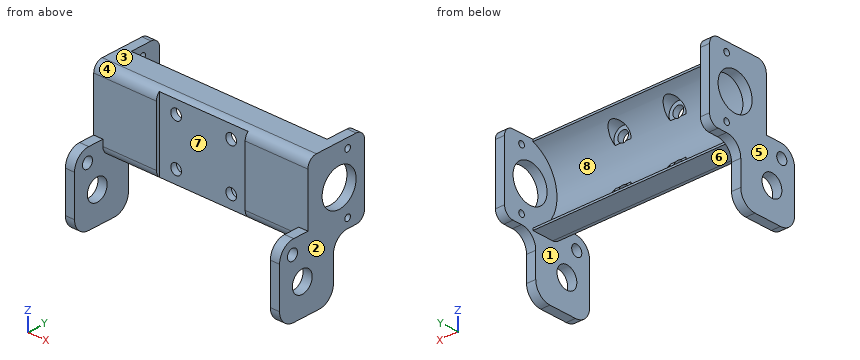
```python
from build123d import *

# Parameters (mm, degrees)
SKETCH1_W            = 70
SKETCH1_H            = 25
BOSS_EXTRUDE1_DEPTH  = 10
SKETCH2_W            = 3
SKETCH2_H            = 25
BOSS_EXTRUDE2_DEPTH  = 10
SKETCH3_R            = 12.5
CUT_EXTRUDE1_DEPTH   = 67
SKETCH4_R            = 3
CUT_EXTRUDE2_DEPTH   = 41.868692174
SKETCH5_R            = 1.75
CUT_EXTRUDE3_DEPTH   = 41.868692259
SKETCH6_W            = 29
SKETCH6_H            = 13
CUT_EXTRUDE4_DEPTH   = 1
SKETCH9_W            = 25
SKETCH9_H            = 20
BOSS_EXTRUDE3_DEPTH  = 3
SKETCH8_R            = 6
SKETCH8_R_2          = 1
CUT_EXTRUDE6_DEPTH   = 74.866433513
FILLET1_R            = 3
SKETCH10_W           = 23
SKETCH10_H           = 19
BOSS_EXTRUDE4_DEPTH  = 3
FILLET2_R            = 5
SKETCH11_R           = 3.5
CUT_EXTRUDE7_DEPTH   = 79.931932702
FILLET2_OF_MIRROR2_R = 5
FILLET3_R            = 5
FILLET4_R            = 3
SKETCH12_R           = 1.784400781
CUT_EXTRUDE8_DEPTH   = 79.931932702


# Some blends are built 0.0001 mm under size
with BuildPart() as part:
    # Sketch1 → Boss-Extrude1 (new body)
    with BuildSketch(Plane(origin=(0, 0, 0), x_dir=(1, 0, 0), z_dir=(0, 1, 0))):
        Rectangle(SKETCH1_W, SKETCH1_H)
    extrude(amount=BOSS_EXTRUDE1_DEPTH)

    # Sketch2 → Boss-Extrude2 (add)
    with BuildSketch(Plane(origin=(0, 10, 0), x_dir=(1, 0, 0), z_dir=(0, 1, 0))):
        with Locations((-33.5, 0)):
            Rectangle(SKETCH2_W, SKETCH2_H)
    extrude(amount=BOSS_EXTRUDE2_DEPTH)

    # Sketch3 → Cut-Extrude1 (cut)
    with BuildSketch(Plane(origin=(35, 0, 0), x_dir=(0, 0, -1), z_dir=(1, 0, 0))):
        with Locations((0, 14)):
            Circle(SKETCH3_R)
    extrude(amount=-CUT_EXTRUDE1_DEPTH, mode=Mode.SUBTRACT)

    # Sketch4 → Cut-Extrude2 (cut, through all)
    with BuildSketch(Plane(origin=(0, 3, 0), x_dir=(1, 0, 0), z_dir=(0, 1, 0))):
        with Locations((-9, 7.5)):
            Circle(SKETCH4_R)
        with Locations((9, 7.5)):
            Circle(SKETCH4_R)
    cut_extrude2 = extrude(amount=CUT_EXTRUDE2_DEPTH, mode=Mode.SUBTRACT)

    # Sketch5 → Cut-Extrude3 (cut, through all)
    with BuildSketch(Plane(origin=(0, 3, 0), x_dir=(1, 0, 0), z_dir=(0, 1, 0))):
        with Locations(Location((-9, 7.5, 0), (0, 0, 270))):
            Circle(SKETCH5_R)
        with Locations(Location((9, 7.5, 0), (0, 0, 270))):
            Circle(SKETCH5_R)
    cut_extrude3 = extrude(amount=-CUT_EXTRUDE3_DEPTH, mode=Mode.SUBTRACT)

    # Sketch6 → Cut-Extrude4 (cut)
    with BuildSketch(Plane.XZ):
        with Locations((0, -6)):
            Rectangle(SKETCH6_W, SKETCH6_H)
    cut_extrude4 = extrude(amount=-CUT_EXTRUDE4_DEPTH, mode=Mode.SUBTRACT)

    # Mirror1: Cut-Extrude2, Cut-Extrude3, Cut-Extrude4 across plane
    add(cut_extrude2.mirror(Plane.XY), mode=Mode.SUBTRACT)
    add(cut_extrude3.mirror(Plane.XY), mode=Mode.SUBTRACT)
    add(cut_extrude4.mirror(Plane.XY), mode=Mode.SUBTRACT)

    # Sketch9 → Boss-Extrude3 (add)
    with BuildSketch(Plane(origin=(35, 0, 0), x_dir=(0, 0, -1), z_dir=(1, 0, 0))):
        with Locations((0, 10)):
            Rectangle(SKETCH9_W, SKETCH9_H)
    extrude(amount=-BOSS_EXTRUDE3_DEPTH)

    # Sketch8 → Cut-Extrude6 (cut, through all)
    with BuildSketch(Plane.ZY.offset(35)):
        with Locations((0, 11)):
            Circle(SKETCH8_R)
        with Locations((-9.5, 14)):
            Circle(SKETCH8_R_2)
        with Locations((9.5, 14)):
            Circle(SKETCH8_R_2)
    extrude(amount=-CUT_EXTRUDE6_DEPTH, mode=Mode.SUBTRACT)

    # Fillet1
    fillet1_edges = [part.edges().sort_by_distance(p)[0] for p in [
        (33.5, 20, 12.5),
        (33.5, 20, -12.5),
        (-33.5, 20, 12.5),
        (-33.5, 20, -12.5),
    ]]
    fillet(fillet1_edges, radius=FILLET1_R)

    # Sketch10 → Boss-Extrude4 (add)
    with BuildSketch(Plane(origin=(35, 0, 0), x_dir=(0, 0, -1), z_dir=(1, 0, 0))):
        with Locations((19, -0.5)):
            Rectangle(SKETCH10_W, SKETCH10_H)
    boss_extrude4 = extrude(amount=-BOSS_EXTRUDE4_DEPTH)

    # Fillet2
    fillet2_edges = [part.edges().sort_by_distance(p)[0] for p in [
        (33.5, -10, -7.5),
        (33.5, 9, -30.5),
        (33.5, -10, -30.5),
    ]]
    fillet(fillet2_edges, radius=FILLET2_R)

    # Sketch11 → Cut-Extrude7 (cut, through all)
    with BuildSketch(Plane(origin=(35, 0, 0), x_dir=(0, 0, -1), z_dir=(1, 0, 0))):
        with Locations((20.5, -2)):
            Circle(SKETCH11_R)
    cut_extrude7 = extrude(amount=-CUT_EXTRUDE7_DEPTH, mode=Mode.SUBTRACT)

    # Mirror2: Boss-Extrude4, Cut-Extrude7 across plane
    add(boss_extrude4.mirror(Plane(origin=(0, 0, 0), x_dir=(0, 0, 1), z_dir=(1, 0, 0))))
    add(cut_extrude7.mirror(Plane(origin=(0, 0, 0), x_dir=(0, 0, 1), z_dir=(1, 0, 0))), mode=Mode.SUBTRACT)

    # Fillet2 of Mirror2
    fillet2_of_mirror2_edges = [part.edges().sort_by_distance(p)[0] for p in [
        (-33.5, -10, -7.5),
        (-33.5, 9, -30.5),
        (-33.5, -10, -30.5),
    ]]
    fillet(fillet2_of_mirror2_edges, radius=FILLET2_OF_MIRROR2_R)

    # Fillet3
    # the kernel refuses this fillet: 5 mm, written as the material it adds along each edge
    with BuildSketch(Plane(origin=(35, 9, -12.5), x_dir=(0, 1, 0), z_dir=(-1, 0, 0)), Plane(origin=(-35, 9, -12.5), x_dir=(0, 0, -1), z_dir=(1, 0, 0))) as fillet3_piece_1:
        with BuildLine():
            CenterArc((FILLET3_R, FILLET3_R), FILLET3_R, 180, 90)
            Line((0, FILLET3_R), (0, 0))
            Line((0, 0), (FILLET3_R, 0))
        make_face()
    extrude(amount=3)

    # Fillet4
    fillet4_edges = [part.edges().sort_by_distance(p)[0] for p in [
        (24.75, 0, 12.5),
        (-23.25, 0, -12.5),
    ]]
    fillet(fillet4_edges, radius=FILLET4_R - 0.0001)  # a hair under: the kernel refuses the full size

    # Sketch12 → Cut-Extrude8 (cut, through all)
    with BuildSketch(Plane.ZY.offset(35)):
        with Locations((-11.755294266, -5.460778231)):
            Circle(SKETCH12_R)
    extrude(amount=-CUT_EXTRUDE8_DEPTH, mode=Mode.SUBTRACT)


solid = part.part
```
Design review of the part built by this model. Coordinates are the model's own, in mm. Face numbers are marked on the shaded views. A direction names the side the tool comes from. Give positions to 0.01 mm unless a question says otherwise; leave off trailing zeros. Loops run counter-clockwise (first coordinate to the right, second up) from the corner with the lowest first, then second, coordinate; pieces in that order, holes last. Notation, with made-up numbers: (42.5, 61.5) -> (101.5, 61.5) arc R29 ccw to (101.5, 87.5) -> close; hole circle Ø11 at (22, -30). An arc over 180 degrees is marked (long way). Write each question's results on one line, items separated by ' | '.
Q1. For pin 1 Ø6 at (x, z) = (-12, -11.5) entering from +Y; pin 2 Ø10 at (x, y) = (-3.5, 5.5) entering from -Z; pin 3 Ø15 at (x, z) = (21, 3) entering from -Y, all flat-tipped, find the tip position at first contact; note any pin that passes through.
Reply:
pin 1: stops at y = 10 | pin 2: stops at z = -12.5 | pin 3: stops at y = 0
Q2. Take a section at D-D, the plane y = -2. Write out the cut boundary in (x, z), plus the area to 3 significant figures.
Reply:
outline: (-35, -30.5) -> (-32, -30.5) -> (-32, -24) -> (-35, -24) -> close; (-35, -17) -> (-32, -17) -> (-32, -7.5) -> (-35, -7.5) -> close; (32, -30.5) -> (35, -30.5) -> (35, -24) -> (32, -24) -> close; (32, -17) -> (35, -17) -> (35, -7.5) -> (32, -7.5) -> close | area: 96.0 mm²
Q3. Wall thickness on L1, parallel to X at y = 2.2, z = 7.5; L2, parallel to Z at x = -9, y = 4.45; L3, parallel to X at y = 8.25, z = -27.5: over which ranges is each line inside the solid? List them lowest first.
Reply:
L1: x = -35 to -10.75, -7.25 to 7.25, 10.75 to 35 | L2: z = -12.5 to -10.5, 10.5 to 12.5 | L3: x = -35 to -32, 32 to 35
Q4. The part is to be moulded in two halves that separate along Z. For the marked faces 1, 2 and 3, say which applies: +Z half, -Z half, draft (parallel to the pull), parting line (faces both ways), or undercut.
Reply:
face 1: undercut | face 2: draft | face 3: +Z half
Q5. Take a section at C-C, the plane z = -20.5. Write out the cut boundary in (x, y).
Reply:
outline: (-35, -10) -> (-32, -10) -> (-32, -5.5) -> (-35, -5.5) -> close; (-35, 1.5) -> (-32, 1.5) -> (-32, 9) -> (-35, 9) -> close; (32, -10) -> (35, -10) -> (35, -5.5) -> (32, -5.5) -> close; (32, 1.5) -> (35, 1.5) -> (35, 9) -> (32, 9) -> close
Q6. Take a section at A-A, the plane y = -8. Write out the cut boundary in (x, z).
Reply:
outline: (-35, -29.5) -> (-32, -29.5) -> (-32, -8.5) -> (-35, -8.5) -> close; (32, -29.5) -> (35, -29.5) -> (35, -8.5) -> (32, -8.5) -> close
Q7. Machinability: for the marked faces 4, 5, 6, 7 and 8, which of the approach directions +Z, -Z, +X, -X, +Y, -Y give a long, thin tool a straight path to every point of the face, cutting with its end or side? Answer none if there is none.
Reply:
face 4: +Z, +X, -X, -Y | face 5: +Z, -Z, -X, +Y, -Y | face 6: -Z, +Y, -Y | face 7: +Z, -Z, -Y | face 8: +Y
Q8. Take a section at B-B, the plane z = 7.5. Write out the cut boundary in (x, y), plus the area to 3 significant figures.
Reply:
outline: (-35, 0) -> (-14.5, 0) -> (-14.5, 1) -> (-10.75, 1) -> (-10.75, 3) -> (-12, 3) -> (-12, 4) -> (-32, 4) -> (-32, 20) -> (-35, 20) -> close; (-7.25, 1) -> (7.25, 1) -> (7.25, 3) -> (6, 3) -> (6, 4) -> (-6, 4) -> (-6, 3) -> (-7.25, 3) -> close; (10.75, 1) -> (14.5, 1) -> (14.5, 0) -> (35, 0) -> (35, 20) -> (32, 20) -> (32, 4) -> (12, 4) -> (12, 3) -> (10.75, 3) -> close | area: 321 mm²
